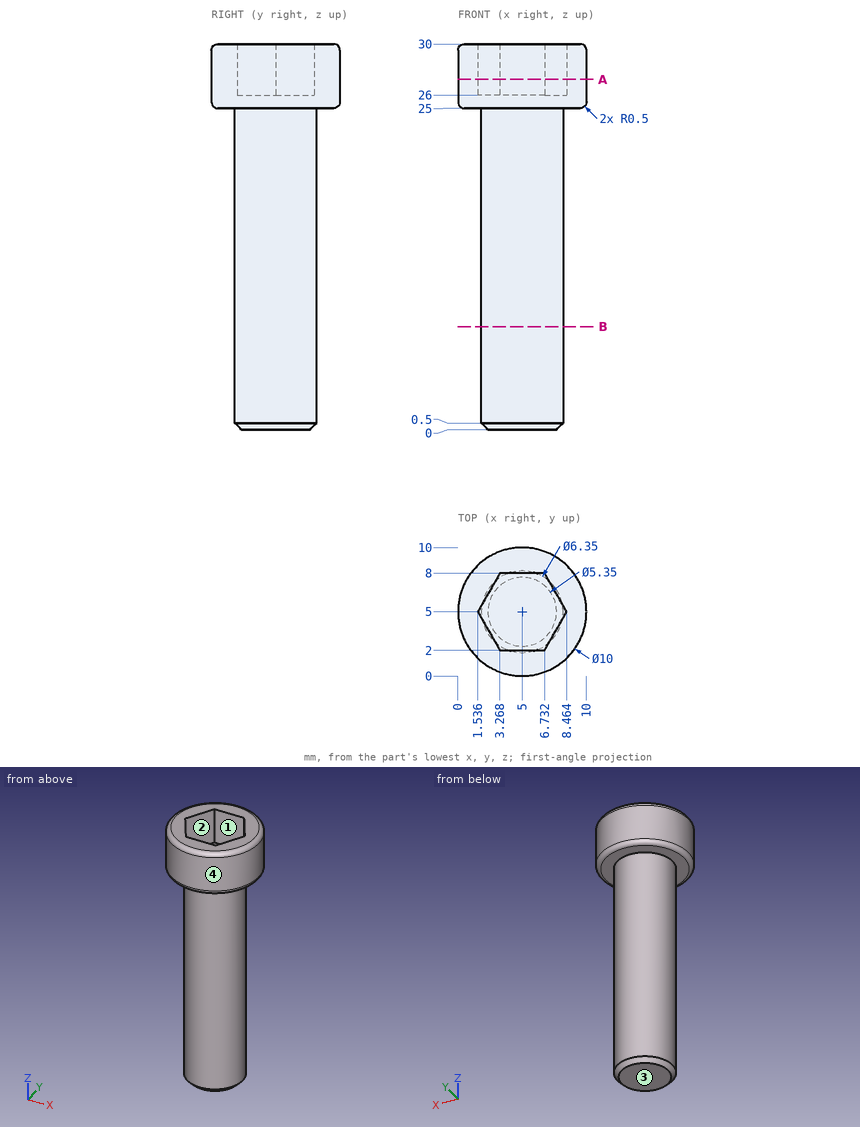
Could you check a few things on this drawing? It's one solid part, dimensions in mm from its lowest x, y, z. Round coordinates to 2 decimals unless told otherwise and drop trailing zeros. Write each loop counter-clockwise with the first axis right and the second up, starting at its lowest first coordinate (ties: lowest second). Pieces come first, ordered by that corner, then holes.
Q1. If we section it at B-B on z = 8: Write out the boundary of the cut face in (x, y) (3 decimals).
Q2. If we mould it in two halves opening along X, with no side actions, what happens to the marked faces 1, 2, 3 and 4? For each: +X half, -X half, draft (parallel to the pull), parting line (faces both ways), or undercut.
Q3. Will these pins go through, and if not, where does the flat tip stop? P1, Ø3, axis at x = 5.5, y = 4, coming from the +Z side; P2, Ø1, axis at y = 3.5, z = 21, coming from the +X side; P3, Ø3, axis at y = 8.5, z = 15.5, coming from the +X side; P4, Ø1, axis at x = 9, z = 8.5, coming from the -Y side.
Q4. If we section it at A-A on z = 27.25: Write out the boundary of the cut face in (x, y).
Q5. Please list where these lines run through material, in increasing order: probe 1 along Z at (x, y) = (7, 8); probe 2 along Y at (x, z) = (5.5, 26.5) (3 decimals); probe 3 along Y at (x, z) = (4, 27.25).
Answer below:
1. outline: circle Ø6.35 at (5, 5)
2. face 1: undercut
2. face 2: undercut
2. face 3: draft
2. face 4: parting line
3. P1: stops at z = 26
3. P2: stops at x = 8.01
3. P3: stops at x = 7.47
3. P4: passes through
4. outline: circle Ø10 at (5, 5); hole (1.54, 5) - (3.27, 2) - (6.73, 2) - (8.46, 5) - (6.73, 8) - (3.27, 8) - close
5. probe 1: z = 25 to 30
5. probe 2: y = 0.025 to 2, 8 to 9.975
5. probe 3: y = 0.1 to 2, 8 to 9.9
